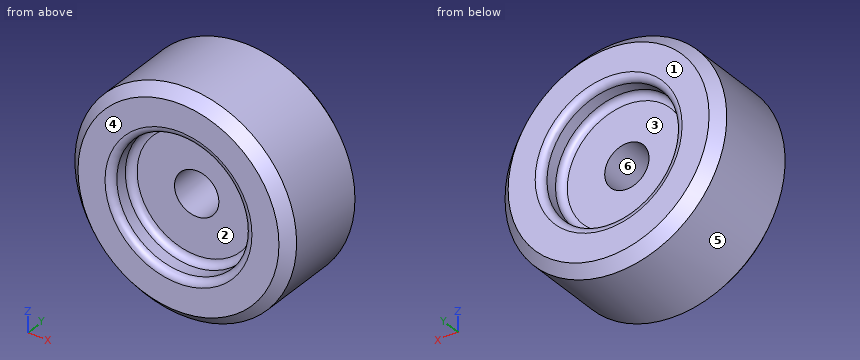
```python
from build123d import *

# Parameters (mm, degrees)
F0_R     = 48
F0_R_2   = 16
F1_DEPTH = 18.75
F0_R_3   = 80
F2_DEPTH = 37.5
F3_SIZE  = 7.5
F4_R     = 5


with BuildPart() as f1:
    # F0 (on Front) → F1 (new body, symmetric)
    with BuildSketch(Plane.XZ):
        Circle(F0_R)
        Circle(F0_R_2, mode=Mode.SUBTRACT)
    extrude(amount=F1_DEPTH, both=True)

    # F0 (on Front) → F2 (join, symmetric)
    with BuildSketch(Plane.XZ):
        Circle(F0_R_3)
        Circle(F0_R, mode=Mode.SUBTRACT)
    extrude(amount=F2_DEPTH, both=True)

    # F3
    f3_edges = [f1.edges().sort_by_distance(p)[0] for p in [
        (-80, 37.5, 0),
        (-80, -37.5, 0),
    ]]
    chamfer(f3_edges, length=F3_SIZE)

    # F4
    f4_edges = [f1.edges().sort_by_distance(p)[0] for p in [
        (-48, -37.5, 0),
        (-48, 37.5, 0),
        (-48, 18.75, 0),
        (-48, -18.75, 0),
    ]]
    fillet(f4_edges, radius=F4_R)


solid = f1.part
```
The listing builds one solid part. Answer for the finished solid, in the listing's coordinates (mm). Face numbers are marked on the shaded views. A direction names the side the tool comes from. Coordinates: 2 decimals unless noted, no trailing zeros. Write each loop counter-clockwise with the first axis right and the second up, starting at its lowest first coordinate (ties: lowest second). Pieces come first, ordered by that corner, then holes.
Q1. Section D-D, the plane y = 28 is taken. Write down the section's boundary in (x, z).
Returned:
outline: circle Ø160 at (0, 0); hole circle Ø96 at (0, 0)
Q2. Section A-A, the plane z = 0 is taken. Write down the section's boundary in (x, y).
Returned:
outline: (-80, -30) - (-72.5, -37.5) - (-53, -37.5) arc R5 ccw to (-48, -32.5) - (-48, -23.75) arc R5 cw to (-43, -18.75) - (-16, -18.75) - (-16, 18.75) - (-43, 18.75) arc R5 cw to (-48, 23.75) - (-48, 32.5) arc R5 ccw to (-53, 37.5) - (-72.5, 37.5) - (-80, 30) - close; (16, -18.75) - (43, -18.75) arc R5 cw to (48, -23.75) - (48, -32.5) arc R5 ccw to (53, -37.5) - (72.5, -37.5) - (80, -30) - (80, 30) - (72.5, 37.5) - (53, 37.5) arc R5 ccw to (48, 32.5) - (48, 23.75) arc R5 cw to (43, 18.75) - (16, 18.75) - close
Q3. The mould has two halves that part along X. Classify the marked faces 4, 5 and 6: released by +X, released by -X, zero draft, split by the parting line, or undercut.
Returned:
face 4: zero draft
face 5: split by the parting line
face 6: undercut
Q4. Given P1, Ø1, axis at y = -13.5, z = 25, coming from the +X side; P2, Ø6, axis at x = 61, z = -53.5, coming from the +Y side; P3, Ø6, axis at x = 27.5, z = 24.5, coming from the +Y side, each flat-ended and moving along its own axis, determine where each tip first touches the part or whether it passes through.
Returned:
P1: stops at x = 76.16
P2: stops at y = 31.86
P3: stops at y = 18.75
Q5. Which of the six approach directions +Z, -Z, +X, -X, +Y, -Y give full straight-line access (tool end or side, diameter ignored) to the marked faces 1, 2 and 3?
Returned:
face 1: +Z, -Z, +X, -X, +Y
face 2: -Y
face 3: +Y
Q6. Find the intervals of material crossed by line 1 along Z through (x, y) = (0, 27.5); line 2 along X through (y, z) = (-26, -1.5); line 3 along X through (y, z) = (-25, 35), in increasing order.
Returned:
line 1: z = -80 to -48, 48 to 80
line 2: x = -79.99 to -47.98, 47.98 to 79.99
line 3: x = -71.94 to -32.85, 32.85 to 71.94
Q7. Section B-B, the plane x = 0 is taken. Write down the section's boundary in (y, z).
Returned:
outline: (-37.5, -72.5) - (-30, -80) - (30, -80) - (37.5, -72.5) - (37.5, -53) arc R5 ccw to (32.5, -48) - (23.75, -48) arc R5 cw to (18.75, -43) - (18.75, -16) - (-18.75, -16) - (-18.75, -43) arc R5 cw to (-23.75, -48) - (-32.5, -48) arc R5 ccw to (-37.5, -53) - close; (-37.5, 53) arc R5 ccw to (-32.5, 48) - (-23.75, 48) arc R5 cw to (-18.75, 43) - (-18.75, 16) - (18.75, 16) - (18.75, 43) arc R5 cw to (23.75, 48) - (32.5, 48) arc R5 ccw to (37.5, 53) - (37.5, 72.5) - (30, 80) - (-30, 80) - (-37.5, 72.5) - close
Q8. Section C-C, the plane y = -14 is taken. Write down the section's boundary in (x, z).
Returned:
outline: circle Ø160 at (0, 0); hole circle Ø32 at (0, 0)
